Autodesk Inventor part; units mm, degrees
ref_plane "YZ Plane" through (0, 0, 0) normal (1, 0, 0) x (0, 1, 0)
ref_plane "XZ Plane" through (0, 0, 0) normal (0, 1, 0) x (-1, 0, 0)
ref_plane "XY Plane" through (0, 0, 0) normal (0, 0, 1) x (1, 0, 0)
sketch "Sketch1" plane through (0, 0, 0) normal (0, 0, 1) x (1, 0, 0)
  line L0 (0, 0) -> (2.5, 0)
  line L1 (2.5, 0) -> (2.5, 25)
  line L2 (2.5, 25) -> (-2.5, 25)
  line L3 (-2.5, 25) -> (-2.5, 0)
  circle A0 centre (0, 0) radius 8.5
  line L4 (0, 25) -> (8.5, 25) construction
  circle A1 centre (0, 25) radius 8.5
  line L5 (-8.5, 0) -> (-8.5, 25)
  line L6 (8.5, 25) -> (8.5, 0)
  line L7 (0, 25) -> (8.5, 25)
  line L8 (0, 25) -> (-8.5, 16.5)
  line L9 (0, 25) -> (12.0208, 25) construction
  line L10 (0, 0) -> (8.5, 0)
  line L11 (0, 0) -> (-8.5, 8.5)
  line L12 (0, 0) -> (12.0208, 0) construction
  dimension "d9" = 17
  dimension "d1" = 2.5
  dimension "d2" = 25
  dimension "d3" = 5
  dimension "d5" = 17
  dimension "d10" = 2.5
  dimension "d11" = 0
  dimension "d12" = 135
  dimension "d13" = 135
extrude "Extrusion1" add sketch "Sketch1" along normal blind 20 contours L11 L3 A0 L1 L0 | L1 A0 L10 | L11 A0 L3 | A0 L3 A1 L1 | L1 A1 L6 A0 | A0 L11 L5 L8 A1 L3 | A1 L3 L8 L2 L1 | L1 L7 A1 | A1 L8 L3
sketch "Sketch2" plane through (0, 0, 0) normal (0, 0, -1) x (-1, 0, 0)
  line L0 (0, 0) -> (-8.5, 0)
  line L1 (0, 0) -> (0, 8)
  circle A0 centre (0, 8) radius 2.5
  line L2 (8.5, 8.5) -> (0, 0)
  line L3 (0, 0) -> (-1.5, 0)
  line L4 (-1.5, 0) -> (-1.5, 8)
  line L5 (-1.5, 8) -> (1.5, 8)
  line L6 (1.5, 8) -> (1.5, 0)
  line L7 (1.5, 0) -> (0, 0)
  line L8 (0, 25) -> (8.5, 16.5)
  line L9 (0, 25) -> (0, 17)
  line L10 (0, 17) -> (-1.5, 17)
  line L11 (-1.5, 17) -> (-1.5, 25)
  line L12 (-8.5, 25) -> (0, 25)
  line L13 (0, 17) -> (1.5, 17)
  line L14 (1.5, 17) -> (1.5, 25)
  line L15 (1.5, 25) -> (0, 25)
  circle A1 centre (0, 17) radius 2.5
  point P0 (1.5, 45)
  point P1 (-1.5, 19)
  point P2 (1.5, 19)
  point P3 (-1.5, 6)
  point P4 (1.5, 6)
  dimension "d16" = 8
  dimension "d17" = 5
  dimension "d18" = 1.5
  dimension "d19" = 3
  dimension "d20" = 8
  dimension "d21" = 1.5
  dimension "d22" = 1.5
  dimension "d23" = 5
extrude "Extrusion2" cut sketch "Sketch2" against normal through all
fillet "Fillet1" radius 8 4 edges at (8.5, 12.5, 0) (8.5, 12.5, 20) (-8.5, 12.5, 0) (-8.5, 12.5, 20)
sketch "Sketch4" plane through (1.5, 0, 0.0627) normal (0, -1, 0) x (1, 0, 0)
  line L0 (-10, 7.9373) -> (-10, 11.9373)
  line L1 (-10, 9.9373) -> (-8, 9.9373)
  circle A0 centre (-8, 9.9373) radius 1
  point P0 (-1.5, -0.0627)
  dimension "d31" = 2
  dimension "d32" = 2
extrude "Extrusion4" cut sketch "Sketch4" against normal through all
properties part number "index_f2"
Source: CAD feature listing. Evaluate the final solid. Frame: model axes, mm. A direction names the side the tool comes from. Round coordinates to 2 decimals unless told otherwise and drop trailing zeros. Loops run counter-clockwise (first coordinate to the right, second up) from the corner with the lowest first, then second, coordinate; pieces in that order, holes last.
Q1. Section B-B, the plane y = 12.75. Return loops of the section in (x, z), plus the area to 3 significant figures.
Q2. Section C-C, the plane y = 9.5. Return loops of the section in (x, z).
Q3. Section A-A, the plane z = 10. Return loops of the section in (x, y), plus the area to 3 significant figures.
Q4. Section D-D, the plane x = -6.5. Return loops of the section in (y, z), plus the area to 3 significant figures.
Q5. Mould query, pull axis X, two halves, no side actions, for faces 4 (the face through (-8.5, 12, 10)), 5 (the face through (0, 13, 0)), 6 (the face through (1.5, 3, 10)), 7 (the face through (8.5, 13, 10)). Classes: pulls with the +X half, pulls with the -X half, needs draft (parallel to the pull), parting line crosses it, or undercut.
Q6. Ray query, line 1 (X direction, y = 11.5, z = 10); line 2 (Y direction, x = 2, z = 15); line 3 (Y direction, x = -2, z = 11.5). Return the intervals inside material, ascending.
Q7. First-contact query: P1, Ø1.2, axis at x = -6.5, z = 10, coming from the +Y side; P2, Ø6.5, axis at y = 2, z = 9, coming from the -X side; P3, Ø2, axis at y = 22, z = 3, coming from the +X side; P4, Ø1.3, axis at y = 21.5, z = 6, coming from the +X side. Flat tips, straight axial feed; report the tip coordinate or a pass-through.
Q8. Access query for faces 1 (the face through (-1.5, 21, 10)), 2 (the face through (0, 13, 20)), 3 (the face through (-1.5, 4, 10)). Directions: +Z, -Z, +X, -X, +Y, -Y. A direction counts if a zero-diameter tool reaches every point of the face in a straight line with its end or side. Return the directions, or none.
Solutions:
1. outline: (-8.5, 8) arc R8 ccw to (-0.5, 0) - (0.5, 0) arc R8 ccw to (8.5, 8) - (8.5, 12) arc R8 ccw to (0.5, 20) - (-0.5, 20) arc R8 ccw to (-8.5, 12) - close; hole circle Ø2 at (-6.5, 10)
1. area: 282 mm2
2. outline: (-8.5, 8) arc R8 ccw to (-2, 0.14) - (-2, 19.86) arc R8 ccw to (-8.5, 12) - close; (2, 0.14) arc R8 ccw to (8.5, 8) - (8.5, 12) arc R8 ccw to (2, 19.86) - close; hole circle Ø2 at (-6.5, 10)
3. outline: (-8.5, 8.5) - (-7.5, 7.5) - (-7.5, 17.5) - (-8.5, 16.5) - close; (-5.5, 5.5) - (-1.5, 1.5) - (-1.5, 6) arc R2.5 cw (long way) to (1.5, 6) - (1.5, 0) - (8.5, 0) - (8.5, 25) - (1.5, 25) - (1.5, 19) arc R2.5 cw (long way) to (-1.5, 19) - (-1.5, 23.5) - (-5.5, 19.5) - close
3. area: 258 mm2
4. outline: (6.5, 2.71) - (18.5, 2.71) - (18.5, 9) - (6.5, 9) - close; (6.5, 11) - (18.5, 11) - (18.5, 17.29) - (6.5, 17.29) - close
4. area: 151 mm2
5. face 4: pulls with the -X half
5. face 5: needs draft
5. face 6: undercut
5. face 7: pulls with the +X half
6. line 1: x = -8.5 to -7.5, -5.5 to 8.5
6. line 2: y = 0 to 6.5, 9.5 to 15.5, 18.5 to 25
6. line 3: y = 2 to 6.5, 9.5 to 15.5, 18.5 to 23
7. P1: passes through
7. P2: stops at x = -5.25
7. P3: stops at x = 7.43
7. P4: stops at x = 8.39
8. face 1: +Z, -Z, +Y
8. face 2: +Z, +X, -X, +Y, -Y
8. face 3: +Z, -Z, -Y
